Here's how the part is built. I have some questions about the finished solid (model axes, mm). A direction names the side the tool comes from. Give positions to 0.01 mm unless a question says otherwise; leave off trailing zeros. Write each loop counter-clockwise with the first axis right and the second up, starting at its lowest first coordinate (ties: lowest second). Pieces come first, ordered by that corner, then holes. Notation, with made-up numbers: (-29.75, -24.5) -> (5.25, -24.5) arc R13 ccw to (5.25, -5.5) -> close; hole circle Ø9 at (33, 55.5). An arc over 180 degrees is marked (long way). Put each result on its own line as item: value. Start each with the question number.
from build123d import *
from build123d.topology import SkipClean

# Parameters (mm, degrees)
BOSS_EXTRU_1_DEPTH           = 10
ENL_V_MAT_EXTRU_1_DEPTH      = 29.854594898
ENL_V_MAT_EXTRU_1_DEPTH_BACK = 29.854594898
ESQUISSE2_R                  = 2.5
ENL_V_START                  = 4
ESQUISSE3_R                  = 6
ENL_V_MAT_EXTRU_2_DEPTH      = 25.390139133
ESQUISSE5_W                  = 1.5
ESQUISSE5_H                  = 4
ENL_V_MAT_EXTRU_3_DEPTH      = 30.220241272
BOSS_EXTRU_2_REACH           = 35.257
ENL_V_START_2                = -20
ESQUISSE7_R                  = 1.2
ESQUISSE7_R_2                = 6
ENL_V_MAT_EXTRU_4_DEPTH      = 20
CONG_1_START                 = -10
CONG_1_DEPTH                 = 20
CONG_1_2_DEPTH               = 20
CONG_1_START_2               = 5.75277665
CONG_1_3_OUTLINE_R           = 6
CONG_1_3_DEPTH               = 28.24722335
CONG_1_START_3               = -1.5
CONG_1_4_DEPTH               = 7.669577456
CONG_1_5_DEPTH               = 2.598076411
CONG_1_START_4               = 22.494446401
CONG_1_6_DEPTH               = 2.598076411
CONG_1_7_DEPTH               = 20


with BuildPart() as part:
    # Esquisse1 → Boss.-Extru.1 (new, symmetric)
    with BuildSketch(Plane(origin=(0, 0, 0), x_dir=(1, 0, 0), z_dir=(0, 1, 0))):
        Polygon((2.35, 0), (9, 0), (9, -2), (1, -6.618802154), (1, -25), (-9, -25), (-9, 0), (-2.35, 0), (-2.35, 1.5), (2.35, 1.5), align=None)
    extrude(amount=BOSS_EXTRU_1_DEPTH, both=True)

    # Esquisse2 → Enlèv. mat.-Extru.1 (cut, two sides: drawn at the far end of the back side and taken through both)
    with BuildSketch(Plane(origin=(-1.372446517, 0, 0), x_dir=(1, 0, 0), z_dir=(0, 0, 1)).offset(-ENL_V_MAT_EXTRU_1_DEPTH_BACK)):
        with Locations(Location((1.372446517, 0, 0), (0, 0, 340.051556411))):
            Circle(ESQUISSE2_R)
    extrude(amount=ENL_V_MAT_EXTRU_1_DEPTH + ENL_V_MAT_EXTRU_1_DEPTH_BACK, mode=Mode.SUBTRACT)

    # Esquisse3 → Enlèv. mat.-Extru.2 (cut, through all)
    with BuildSketch(Plane.XY.offset(ENL_V_START)):
        Circle(ESQUISSE3_R)
    extrude(amount=ENL_V_MAT_EXTRU_2_DEPTH, mode=Mode.SUBTRACT)

    # Esquisse5 → Enlèv. mat.-Extru.3 (cut, through all)
    with BuildSketch(Plane.ZY.offset(2.35)):
        with Locations((-0.75, 0)):
            Rectangle(ESQUISSE5_W, ESQUISSE5_H)
    extrude(amount=-ENL_V_MAT_EXTRU_3_DEPTH, mode=Mode.SUBTRACT)

    # Boss.-Extru.2: up to this face of the body (flat: up to its plane)
    boss_extru_2_end = Plane(part.part.faces().sort_by_distance((-2.923443816, -10, 10.980550797))[0])
    # Esquisse6 → Boss.-Extru.2 (add, up to the picked face)
    with BuildSketch(Plane(origin=(0, 10, 0), x_dir=(1, 0, 0), z_dir=(0, 1, 0)), mode=Mode.PRIVATE) as boss_extru_2_sk1:
        Polygon((-9, -18.452994616), (5.803847577, -27), (13, -27), (13, -33), (-3.803847577, -33), (-9, -30), align=None)
    boss_extru_2_tool1 = split(extrude(boss_extru_2_sk1.sketch, amount=-BOSS_EXTRU_2_REACH, mode=Mode.PRIVATE), bisect_by=boss_extru_2_end, keep=Keep.BOTH, mode=Mode.PRIVATE)
    add(boss_extru_2_tool1.solids().sort_by(Axis((0.338478, 10, 27.943024), (0, -1, 0)))[0])

    # Esquisse7 → Enlèv. mat.-Extru.4 (cut)
    with BuildSketch(Plane.XY.offset(33).offset(ENL_V_START_2)):
        with Locations((10, 0)):
            Circle(ESQUISSE7_R)
        with Locations(Location((0, 0, 0), (0, 0, 230.656026391))):
            Circle(ESQUISSE7_R_2)
    extrude(amount=ENL_V_MAT_EXTRU_4_DEPTH, mode=Mode.SUBTRACT)

    # Congé1: read off the stored shape, not the designer's step
    # Congé1 outline → Congé1 (cut)
    with BuildSketch(Plane(origin=(0, 0, 0), x_dir=(1, 0, 0), z_dir=(0, 1, 0)).offset(CONG_1_START)):
        with BuildLine():
            Line((-9, -30), (-7.5, -30.866025404))
            ThreePointArc((-7.5, -30.866025404), (-8.598076211, -29.767949192), (-9, -28.267949192))
            Line((-9, -28.267949192), (-9, -30))
        make_face()
    extrude(amount=CONG_1_DEPTH, mode=Mode.SUBTRACT)

    # Cong_1 2 outline → Cong_1 2 (add)
    with BuildSketch(Plane(origin=(0, 0, 0), x_dir=(1, 0, 0), z_dir=(0, 1, 0)).offset(CONG_1_START)):
        with BuildLine():
            Line((5.803847577, -27), (6.607695155, -27))
            ThreePointArc((6.607695155, -27), (5.83123802, -26.897777479), (5.107695155, -26.598076211))
            Line((5.107695155, -26.598076211), (5.803847577, -27))
        make_face()
    extrude(amount=CONG_1_2_DEPTH)

    # Cong_1 3 outline → Cong_1 3 (cut)
    with BuildSketch(Plane.XY.offset(CONG_1_START_2)):
        with BuildLine():
            Line((-9, 10), (-9, 7))
            ThreePointArc((-9, 7), (-8.121320344, 9.121320344), (-6, 10))
            Line((-6, 10), (-9, 10))
        make_face()
        with BuildLine():
            ThreePointArc((-6, -10), (-8.121320344, -9.121320344), (-9, -7))
            Line((-9, -7), (-9, -10))
            Line((-9, -10), (-6, -10))
        make_face()
        Circle(CONG_1_3_OUTLINE_R)
        with BuildLine():
            Line((13, 10), (10, 10))
            ThreePointArc((10, 10), (12.121320344, 9.121320344), (13, 7))
            Line((13, 7), (13, 10))
        make_face()
        with BuildLine():
            ThreePointArc((13, -7), (12.121320344, -9.121320344), (10, -10))
            Line((10, -10), (13, -10))
            Line((13, -10), (13, -7))
        make_face()
    extrude(amount=CONG_1_3_DEPTH, mode=Mode.SUBTRACT)

    # Cong_1 4 outline → Cong_1 4 (cut)
    with BuildSketch(Plane.XY.offset(CONG_1_START_3)):
        with BuildLine():
            Line((-9, 10), (-9, 7))
            ThreePointArc((-9, 7), (-8.121320344, 9.121320344), (-6, 10))
            Line((-6, 10), (-9, 10))
        make_face()
        with BuildLine():
            ThreePointArc((-6, -10), (-8.121320344, -9.121320344), (-9, -7))
            Line((-9, -7), (-9, -10))
            Line((-9, -10), (-6, -10))
        make_face()
        with BuildLine():
            Line((9, 10), (6, 10))
            ThreePointArc((6, 10), (8.121320344, 9.121320344), (9, 7))
            Line((9, 7), (9, 10))
        make_face()
        with BuildLine():
            ThreePointArc((9, -7), (8.121320344, -9.121320344), (6, -10))
            Line((6, -10), (9, -10))
            Line((9, -10), (9, -7))
        make_face()
    extrude(amount=CONG_1_4_DEPTH, mode=Mode.SUBTRACT)

    # Cong_1 5 outline → Cong_1 5 (add)
    with SkipClean():  # the faces are left unmerged after this step: merging them gives an invalid solid
        with BuildSketch(Plane.XY.offset(CONG_1_START_2)):
            with BuildLine():
                Line((6, 10), (1, 10))
                Line((1, 10), (1, 5.916079783))
                ThreePointArc((1, 5.916079783), (6, 0), (1, -5.916079783))
                Line((1, -5.916079783), (1, -10))
                Line((1, -10), (6, -10))
                ThreePointArc((6, -10), (8.121320344, -9.121320344), (9, -7))
                Line((9, -7), (9, 7))
                ThreePointArc((9, 7), (8.121320344, 9.121320344), (6, 10))
            make_face()
        extrude(amount=CONG_1_5_DEPTH)

    # Cong_1 6 outline → Cong_1 6 (add)
    with SkipClean():  # the faces are left unmerged after this step: merging them gives an invalid solid
        with BuildSketch(Plane.XY.offset(CONG_1_START_4)):
            with BuildLine():
                Line((6, 10), (1, 10))
                Line((1, 10), (1, 5.916079783))
                ThreePointArc((1, 5.916079783), (6, 0), (1, -5.916079783))
                Line((1, -5.916079783), (1, -10))
                Line((1, -10), (6, -10))
                ThreePointArc((6, -10), (8.121320344, -9.121320344), (9, -7))
                Line((9, -7), (9, 7))
                ThreePointArc((9, 7), (8.121320344, 9.121320344), (6, 10))
            make_face()
        extrude(amount=CONG_1_6_DEPTH)

    # Cong_1 7 outline → Cong_1 7 (cut)
    with SkipClean():  # the faces are left unmerged after this step: merging them gives an invalid solid
        with BuildSketch(Plane(origin=(0, 0, 0), x_dir=(1, 0, 0), z_dir=(0, 1, 0)).offset(CONG_1_START)):
            with BuildLine():
                ThreePointArc((-3, -33), (-3.776457135, -32.897777479), (-4.5, -32.598076211))
                Line((-4.5, -32.598076211), (-3.803847577, -33))
                Line((-3.803847577, -33), (-3, -33))
            make_face()
            with BuildLine():
                ThreePointArc((1, -22.494446501), (1.401923789, -23.994446501), (2.5, -25.092522712))
                Line((2.5, -25.092522712), (9, -25.092522812))
                Line((9, -25.092522812), (9, -22.494446401))
                Line((9, -22.494446401), (1, -22.494446501))
            make_face()
            with BuildLine():
                Line((9, -5.75277665), (2.5, -5.75277675))
                ThreePointArc((2.5, -5.75277675), (1.401923789, -6.850852961), (1, -8.350852961))
                Line((1, -8.350852961), (9, -8.350853061))
                Line((9, -8.350853061), (9, -5.75277665))
            make_face()
        extrude(amount=CONG_1_7_DEPTH, mode=Mode.SUBTRACT)


solid = part.part
1) I need wall thicknesses on probe 1 along Y at (x, z) = (0, 25.75); probe 2 along Y at (x, z) = (10, 28.95); probe 3 along X at (y, z) = (0, 1.6). Which ranges of each line are inside material? Lowest first, please.
2) I want a section at B-B, the plane z = 17.5. Write out the boundary of the cut face in (x, y).
3) I want a section at D-D, the plane x = -5.25. Write out the boundary of the cut face in (y, z).
4) Thinking about a two-plate mould opening in Y: for faces 5 (the flat face through (0, -10, 16)), 6 (the flat face through (-2, -2, -1)), 7 (the flat face through (0, 6, -1.5)), 8 (the cylindrical face through (12.1, 9.14, 29.96)), which applies, released by +Y, released by -Y, zero draft, split by the parting line, or undercut?
5) I want a section at C-C, the plane y = 0.5. Write out the boundary of the cut face in (x, z).
6) I'm going to push flat-ended pins straight in: pin 1 Ø1.6 at (y, z) = (-5, -1) entering from -X; pin 2 Ø2 at (x, y) = (-5.5, -1.5) entering from -Z; pin 3 Ø3 at (x, y) = (10.5, -8) entering from -Z. Where does each tip first touch, or does it pass through?
7) Which directions (+Z, -Z, +X, -X, +Y, -Y) give clear straight access to the entire face, cutting with the end or side of a thin tool? Please do faces 1 (the flat face through (1, 8, 15)), 2 (the flat face through (0, -3, 4)), 3 (the flat face through (2.35, 6, -1)), 4 (the flat face through (2, 2, -1)).
8) I want a section at A-A, the plane x = 0. Write out the boundary of the cut face in (y, z).
Established:
1. probe 1: y = -10 to -6, 6 to 10
1. probe 2: y = -10 to -1.2, 1.2 to 10
1. probe 3: x = -9 to -2.5, 2.5 to 9
2. outline: (-9, -7) arc R3 ccw to (-6, -10) -> (1, -10) -> (1, -5.92) arc R6 cw (long way) to (1, 5.92) -> (1, 10) -> (-6, 10) arc R3 ccw to (-9, 7) -> close
3. outline: (-10, 0) -> (10, 0) -> (10, 32.17) -> (2.9, 32.17) -> (2.9, 4) -> (-2.9, 4) -> (-2.9, 32.17) -> (-10, 32.17) -> close
4. face 5: released by -Y
4. face 6: undercut
4. face 7: zero draft
4. face 8: released by +Y
5. outline: (-9, 0) -> (-2.45, 0) -> (-2.45, 4) -> (-5.98, 4) -> (-5.98, 31.74) -> (-7.5, 30.87) arc R3 ccw to (-9, 28.27) -> close; (2.45, 0) -> (9, 0) -> (9, 2) -> (5.54, 4) -> (2.45, 4) -> close; (5.98, 26.93) arc R3 cw to (6.61, 27) -> (8.91, 27) -> (8.91, 33) -> (5.98, 33) -> close; (11.09, 27) -> (13, 27) -> (13, 33) -> (11.09, 33) -> close
6. pin 1: stops at x = -2.35
6. pin 2: stops at z = 0
6. pin 3: stops at z = 27
7. face 1: +X, +Y, -Y
7. face 2: +Z
7. face 3: -Z, +X, +Y, -Y
7. face 4: -Z, +X, -X
8. outline: (-10, -1.5) -> (-2.5, -1.5) -> (-2.5, 4) -> (-6, 4) -> (-6, 33) -> (-10, 33) -> close; (2.5, -1.5) -> (10, -1.5) -> (10, 33) -> (6, 33) -> (6, 4) -> (2.5, 4) -> close
